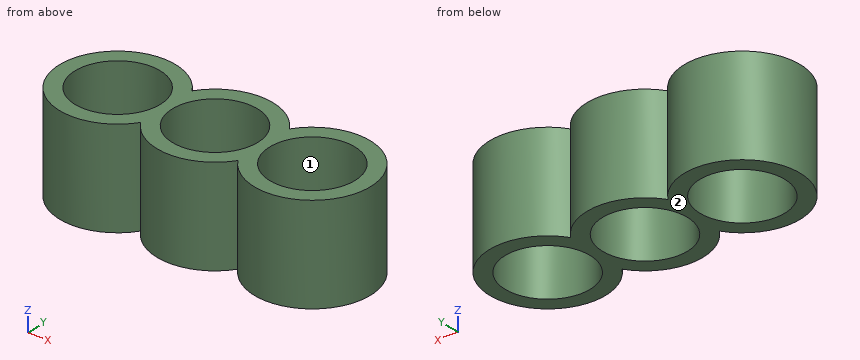
from build123d import *

# Parameters (mm, degrees)
F0_R     = 11
F1_DEPTH = 25


with BuildPart() as f1:
    # F0 (on Top) → F1 (new body)
    with BuildSketch(Plane.XY):
        with BuildLine():
            ThreePointArc((-12.5, 8.291562), (-40, 0), (-12.5, -8.291562))
            ThreePointArc((-12.5, -8.291562), (0, -15), (12.5, -8.291562))
            ThreePointArc((12.5, -8.291562), (40, 0), (12.5, 8.291562))
            ThreePointArc((12.5, 8.291562), (0, 15), (-12.5, 8.291562))
        make_face()
        with Locations((-25, 0)):
            Circle(F0_R, mode=Mode.SUBTRACT)
        with BuildLine():
            ThreePointArc((-11, 0), (0, 11), (11, 0))
            ThreePointArc((11, 0), (0, -11), (-11, 0))
        make_face(mode=Mode.SUBTRACT)
        with Locations((25, 0)):
            Circle(F0_R, mode=Mode.SUBTRACT)
    extrude(amount=F1_DEPTH)


solid = f1.part
Verification items for the finished model (mm, model axes). Face numbers are marked on the shaded views. Round coordinates to 2 decimals unless told otherwise and drop trailing zeros. Order: outer loops, then holes, each group sorted by start corner. A loop starts at its lowest first (then second) coordinate and runs counter-clockwise, first axis right, second up. Notation, with made-up numbers: (-21.5, 71.5) -> (-13.5, 71.5) arc R15 cw to (-13.5, 76.5) -> close; hole circle Ø7 at (-9, -3). An arc over 180 degrees is marked (long way). Put each result on its own line as item: value.
1) Section check D-D (y = 9.5). Record the cut outline in (x, z).
Final values:
outline: (-36.61, 0) -> (-30.55, 0) -> (-30.55, 25) -> (-36.61, 25) -> close; (-19.45, 0) -> (-13.39, 0) -> (-13.39, 25) -> (-19.45, 25) -> close; (-11.61, 0) -> (-5.55, 0) -> (-5.55, 25) -> (-11.61, 25) -> close; (5.55, 0) -> (11.61, 0) -> (11.61, 25) -> (5.55, 25) -> close; (13.39, 0) -> (19.45, 0) -> (19.45, 25) -> (13.39, 25) -> close; (30.55, 0) -> (36.61, 0) -> (36.61, 25) -> (30.55, 25) -> close
2) Section check B-B (z = 17.5). Record the cut outline in (x, y).
Final values:
outline: (-12.5, -8.29) arc R15 ccw to (12.5, -8.29) arc R15 ccw (long way) to (12.5, 8.29) arc R15 ccw to (-12.5, 8.29) arc R15 ccw (long way) to start; hole circle Ø22 at (-25, 0); hole circle Ø22 at (0, 0); hole circle Ø22 at (25, 0)
3) Material ranges on line 1 (X direction, y = -12.5, z = 9.5); line 2 (Y direction, x = -25, z = 19.75); line 3 (X direction, y = 12, z = 11), recorded low to high.
Final values:
line 1: x = -33.29 to -16.71, -8.29 to 8.29, 16.71 to 33.29
line 2: y = -15 to -11, 11 to 15
line 3: x = -34 to -16, -9 to 9, 16 to 34
4) Section check C-C (x = 25). Record the cut outline in (y, z).
Final values:
outline: (-15, 0) -> (-11, 0) -> (-11, 25) -> (-15, 25) -> close; (11, 0) -> (15, 0) -> (15, 25) -> (11, 25) -> close
5) Section check A-A (y = 0). Record the cut outline in (x, z).
Final values:
outline: (-40, 0) -> (-36, 0) -> (-36, 25) -> (-40, 25) -> close; (-14, 0) -> (-11, 0) -> (-11, 25) -> (-14, 25) -> close; (11, 0) -> (14, 0) -> (14, 25) -> (11, 25) -> close; (36, 0) -> (40, 0) -> (40, 25) -> (36, 25) -> close
6) Mould release check, pull along Y, two halves, no side actions. Record for the marked faces 1 and 2: +Y half, -Y half, draft (parallel to the pull), parting line (faces both ways), or undercut.
Final values:
face 1: undercut
face 2: draft
7) Depth check by flat-ended pin: pin 1 (5 mm diameter, centred on y = 4.5, z = 18.5, fed in from -X); pin 2 (2 mm diameter, centred on x = -22, z = 11.5, fed in from -Y); pin 3 (1 mm diameter, centred on x = 28.5, z = 8.5, fed in from +Y). Enter the tip coordinate at first touch or a pass-through.
Final values:
pin 1: stops at x = -39.87
pin 2: stops at y = -14.87
pin 3: stops at y = 14.7
